```python
from build123d import *

# Parameters (mm, degrees)
EXTRUDE_1_DEPTH     = 3
CUT_EXTRUDE_2_REACH = 76.221
SKETCH_2_R          = 2.1
FILLET_1_R          = 2


with BuildPart() as part:
    # 草图1 → 凸台-拉伸1 (new body)
    with BuildSketch(Plane.XY):
        Polygon((-15, 45.229945154), (15, 45.229945154), (50, -29.684017461), (50, -54.770054846), (-50, -54.770054846), (-50, -29.684017461), align=None)
    extrude(amount=EXTRUDE_1_DEPTH)

    # 草图2 → 切除-拉伸2 (cut, up to next)
    with BuildSketch(Plane.XY.offset(3), mode=Mode.PRIVATE) as cut_extrude_2_sk1:
        with Locations((-9, 35.229945154)):
            Circle(SKETCH_2_R)
    cut_extrude_2_tool1 = extrude(cut_extrude_2_sk1.sketch, amount=-CUT_EXTRUDE_2_REACH, mode=Mode.PRIVATE) & part.part
    # 草图2 → 切除-拉伸2 (cut, up to next)
    with BuildSketch(Plane.XY.offset(3), mode=Mode.PRIVATE) as cut_extrude_2_sk2:
        with Locations((9, 35.229945154)):
            Circle(SKETCH_2_R)
    cut_extrude_2_tool2 = extrude(cut_extrude_2_sk2.sketch, amount=-CUT_EXTRUDE_2_REACH, mode=Mode.PRIVATE) & part.part
    # 草图2 → 切除-拉伸2 (cut, up to next)
    with BuildSketch(Plane.XY.offset(3), mode=Mode.PRIVATE) as cut_extrude_2_sk3:
        with Locations((9, 10.229945154)):
            Circle(SKETCH_2_R)
    cut_extrude_2_tool3 = extrude(cut_extrude_2_sk3.sketch, amount=-CUT_EXTRUDE_2_REACH, mode=Mode.PRIVATE) & part.part
    # 草图2 → 切除-拉伸2 (cut, up to next)
    with BuildSketch(Plane.XY.offset(3), mode=Mode.PRIVATE) as cut_extrude_2_sk4:
        with Locations((-9, 10.229945154)):
            Circle(SKETCH_2_R)
    cut_extrude_2_tool4 = extrude(cut_extrude_2_sk4.sketch, amount=-CUT_EXTRUDE_2_REACH, mode=Mode.PRIVATE) & part.part
    # 草图2 → 切除-拉伸2 (cut, up to next)
    with BuildSketch(Plane.XY.offset(3), mode=Mode.PRIVATE) as cut_extrude_2_sk5:
        with Locations((-20, -36.770054846)):
            Circle(SKETCH_2_R)
    cut_extrude_2_tool5 = extrude(cut_extrude_2_sk5.sketch, amount=-CUT_EXTRUDE_2_REACH, mode=Mode.PRIVATE) & part.part
    # 草图2 → 切除-拉伸2 (cut, up to next)
    with BuildSketch(Plane.XY.offset(3), mode=Mode.PRIVATE) as cut_extrude_2_sk6:
        with Locations((-20, -46.770054846)):
            Circle(SKETCH_2_R)
    cut_extrude_2_tool6 = extrude(cut_extrude_2_sk6.sketch, amount=-CUT_EXTRUDE_2_REACH, mode=Mode.PRIVATE) & part.part
    # 草图2 → 切除-拉伸2 (cut, up to next)
    with BuildSketch(Plane.XY.offset(3), mode=Mode.PRIVATE) as cut_extrude_2_sk7:
        with Locations((20, -46.770054846)):
            Circle(SKETCH_2_R)
    cut_extrude_2_tool7 = extrude(cut_extrude_2_sk7.sketch, amount=-CUT_EXTRUDE_2_REACH, mode=Mode.PRIVATE) & part.part
    # 草图2 → 切除-拉伸2 (cut, up to next)
    with BuildSketch(Plane.XY.offset(3), mode=Mode.PRIVATE) as cut_extrude_2_sk8:
        with Locations((20, -36.770054846)):
            Circle(SKETCH_2_R)
    cut_extrude_2_tool8 = extrude(cut_extrude_2_sk8.sketch, amount=-CUT_EXTRUDE_2_REACH, mode=Mode.PRIVATE) & part.part
    # 草图2 → 切除-拉伸2 (cut, up to next)
    with BuildSketch(Plane.XY.offset(3), mode=Mode.PRIVATE) as cut_extrude_2_sk9:
        with Locations((-9, -14.770054846)):
            Circle(SKETCH_2_R)
    cut_extrude_2_tool9 = extrude(cut_extrude_2_sk9.sketch, amount=-CUT_EXTRUDE_2_REACH, mode=Mode.PRIVATE) & part.part
    # 草图2 → 切除-拉伸2 (cut, up to next)
    with BuildSketch(Plane.XY.offset(3), mode=Mode.PRIVATE) as cut_extrude_2_sk10:
        with Locations((9, -14.770054846)):
            Circle(SKETCH_2_R)
    cut_extrude_2_tool10 = extrude(cut_extrude_2_sk10.sketch, amount=-CUT_EXTRUDE_2_REACH, mode=Mode.PRIVATE) & part.part
    # 草图2 → 切除-拉伸2 (cut, up to next)
    with BuildSketch(Plane.XY.offset(3), mode=Mode.PRIVATE) as cut_extrude_2_sk11:
        with Locations((-35, -36.770054846)):
            Circle(SKETCH_2_R)
    cut_extrude_2_tool11 = extrude(cut_extrude_2_sk11.sketch, amount=-CUT_EXTRUDE_2_REACH, mode=Mode.PRIVATE) & part.part
    # 草图2 → 切除-拉伸2 (cut, up to next)
    with BuildSketch(Plane.XY.offset(3), mode=Mode.PRIVATE) as cut_extrude_2_sk12:
        with Locations((-35, -46.770054846)):
            Circle(SKETCH_2_R)
    cut_extrude_2_tool12 = extrude(cut_extrude_2_sk12.sketch, amount=-CUT_EXTRUDE_2_REACH, mode=Mode.PRIVATE) & part.part
    # 草图2 → 切除-拉伸2 (cut, up to next)
    with BuildSketch(Plane.XY.offset(3), mode=Mode.PRIVATE) as cut_extrude_2_sk13:
        with Locations((35, -36.770054846)):
            Circle(SKETCH_2_R)
    cut_extrude_2_tool13 = extrude(cut_extrude_2_sk13.sketch, amount=-CUT_EXTRUDE_2_REACH, mode=Mode.PRIVATE) & part.part
    # 草图2 → 切除-拉伸2 (cut, up to next)
    with BuildSketch(Plane.XY.offset(3), mode=Mode.PRIVATE) as cut_extrude_2_sk14:
        with Locations((35, -46.770054846)):
            Circle(SKETCH_2_R)
    cut_extrude_2_tool14 = extrude(cut_extrude_2_sk14.sketch, amount=-CUT_EXTRUDE_2_REACH, mode=Mode.PRIVATE) & part.part
    # 草图2 → 切除-拉伸2 (cut, up to next)
    with BuildSketch(Plane.XY.offset(3), mode=Mode.PRIVATE) as cut_extrude_2_sk15:
        with BuildLine():
            Line((-20.314527419, 5.727067103), (-20.314527419, -23.770054846))
            ThreePointArc((-20.314527419, -23.770054846), (-20.607420638, -24.477161627), (-21.314527419, -24.770054846))
            Line((-21.314527419, -24.770054846), (-35.09566023, -24.770054846))
            ThreePointArc((-35.09566023, -24.770054846), (-35.939249041, -24.307044527), (-36.001657204, -23.346770682))
            Line((-36.001657204, -23.346770682), (-22.220524392, 6.150351268))
            ThreePointArc((-22.220524392, 6.150351268), (-21.097729095, 6.703283517), (-20.314527419, 5.727067103))
        make_face()
    cut_extrude_2_tool15 = extrude(cut_extrude_2_sk15.sketch, amount=-CUT_EXTRUDE_2_REACH, mode=Mode.PRIVATE) & part.part
    # 草图2 → 切除-拉伸2 (cut, up to next)
    with BuildSketch(Plane.XY.offset(3), mode=Mode.PRIVATE) as cut_extrude_2_sk16:
        with BuildLine():
            Line((36.001657204, -23.346770682), (22.220524392, 6.150351268))
            ThreePointArc((22.220524392, 6.150351268), (21.097729095, 6.703283517), (20.314527419, 5.727067103))
            Line((20.314527419, 5.727067103), (20.314527419, -23.770054846))
            ThreePointArc((20.314527419, -23.770054846), (20.607420638, -24.477161627), (21.314527419, -24.770054846))
            Line((21.314527419, -24.770054846), (35.09566023, -24.770054846))
            ThreePointArc((35.09566023, -24.770054846), (35.939249041, -24.307044527), (36.001657204, -23.346770682))
        make_face()
    cut_extrude_2_tool16 = extrude(cut_extrude_2_sk16.sketch, amount=-CUT_EXTRUDE_2_REACH, mode=Mode.PRIVATE) & part.part
    add(cut_extrude_2_tool1.solids().sort_by_distance((-9, 35.229945, 3))[0], mode=Mode.SUBTRACT)
    add(cut_extrude_2_tool2.solids().sort_by_distance((9, 35.229945, 3))[0], mode=Mode.SUBTRACT)
    add(cut_extrude_2_tool3.solids().sort_by_distance((9, 10.229945, 3))[0], mode=Mode.SUBTRACT)
    add(cut_extrude_2_tool4.solids().sort_by_distance((-9, 10.229945, 3))[0], mode=Mode.SUBTRACT)
    add(cut_extrude_2_tool5.solids().sort_by_distance((-20, -36.770055, 3))[0], mode=Mode.SUBTRACT)
    add(cut_extrude_2_tool6.solids().sort_by_distance((-20, -46.770055, 3))[0], mode=Mode.SUBTRACT)
    add(cut_extrude_2_tool7.solids().sort_by_distance((20, -46.770055, 3))[0], mode=Mode.SUBTRACT)
    add(cut_extrude_2_tool8.solids().sort_by_distance((20, -36.770055, 3))[0], mode=Mode.SUBTRACT)
    add(cut_extrude_2_tool9.solids().sort_by_distance((-9, -14.770055, 3))[0], mode=Mode.SUBTRACT)
    add(cut_extrude_2_tool10.solids().sort_by_distance((9, -14.770055, 3))[0], mode=Mode.SUBTRACT)
    add(cut_extrude_2_tool11.solids().sort_by_distance((-35, -36.770055, 3))[0], mode=Mode.SUBTRACT)
    add(cut_extrude_2_tool12.solids().sort_by_distance((-35, -46.770055, 3))[0], mode=Mode.SUBTRACT)
    add(cut_extrude_2_tool13.solids().sort_by_distance((35, -36.770055, 3))[0], mode=Mode.SUBTRACT)
    add(cut_extrude_2_tool14.solids().sort_by_distance((35, -46.770055, 3))[0], mode=Mode.SUBTRACT)
    add(cut_extrude_2_tool15.solids().sort_by_distance((-25.803132, -13.304968, 3))[0], mode=Mode.SUBTRACT)
    add(cut_extrude_2_tool16.solids().sort_by_distance((25.803132, -13.304968, 3))[0], mode=Mode.SUBTRACT)

    # 圆角1
    fillet_1_edges = [part.edges().sort_by_distance(p)[0] for p in [
        (-15, 45.229945154, 1.5),
        (-50, -29.684017461, 1.5),
        (-50, -54.770054846, 1.5),
        (50, -54.770054846, 1.5),
        (50, -29.684017461, 1.5),
        (15, 45.229945154, 1.5),
    ]]
    fillet(fillet_1_edges, radius=FILLET_1_R)


solid = part.part
```
Geometry check sheet. Reference: the model listing, model coordinates, mm. A direction names the side the tool comes from. Give positions to 0.01 mm unless a question says otherwise; leave off trailing zeros. Write each loop counter-clockwise with the first axis right and the second up, starting at its lowest first coordinate (ties: lowest second). Pieces come first, ordered by that corner, then holes.
1) Section check B-B, the plane x = -9. Record the boundary of the cut face in (y, z), and give its area (3 significant figures).
2) Access from +Z, -Z, +X, -X, +Y, -Y to the whole of each face (thin tool, end or side, straight path). Record for faces 1 (the flat face through (28, -24.77, 2)), 2 (the flat face through (50, -41, 1)).
3) Section check A-A, the plane y = -3.5. Record the boundary of the cut face in (x, z).
4) Section check C-C, the plane x = -28. Record the boundary of the cut face in (y, z).
5) Gauge pin test, flat ends, axial feed: pin 1 (3.5 mm diameter, centred on x = 20, y = -36.77, fed in from -Z); pin 2 (0.9 mm diameter, centred on y = -12, z = 2, fed in from +X); pin 3 (1.5 mm diameter, centred on x = 27.5, z = 2, fed in from +Y); pin 4 (5.5 mm diameter, centred on x = -9, y = 35.23, fed in from +Z). Record the tip position at first contact, or that the pin passes through.
6) Release check for a two-part mould opening along Y. For faces 3 (the flat face through (1, -15, 3)), 4 (the flat face through (-32.915, 6.884, 1.479)), 5 (the cylindrical face through (6.9, -14.7, 1.5)) record: pulls with the +Y half, pulls with the -Y half, needs draft (parallel to the pull), parting line crosses it, or undercut.
7) Section check D-D, the plane z = 2.4. State how many separate pieces and enclosed holes the cut face has, and give its area (3 significant figures).
8) Material ranges on L1, parallel to Y at x = -9, z = 2.65; L2, parallel to X at y = 9.5, z = 1.2; L3, parallel to Y at x = 34.5, z = 2.4, recorded low to high.
Computed:
1. outline: (-54.77, 0) - (-16.87, 0) - (-16.87, 3) - (-54.77, 3) - close; (-12.67, 0) - (8.13, 0) - (8.13, 3) - (-12.67, 3) - close; (12.33, 0) - (33.13, 0) - (33.13, 3) - (12.33, 3) - close; (37.33, 0) - (45.23, 0) - (45.23, 3) - (37.33, 3) - close
1. area: 262 mm2
2. face 1: +Z, -Z
2. face 2: +Z, -Z, +X, +Y, -Y
3. outline: (-37.77, 0) - (-26.73, 0) - (-26.73, 3) - (-37.77, 3) - close; (-20.31, 0) - (20.31, 0) - (20.31, 3) - (-20.31, 3) - close; (26.73, 0) - (37.77, 0) - (37.77, 3) - (26.73, 3) - close
4. outline: (-54.77, 0) - (-24.77, 0) - (-24.77, 3) - (-54.77, 3) - close; (-6.22, 0) - (17.4, 0) - (17.4, 3) - (-6.22, 3) - close
5. pin 1: passes through
5. pin 2: stops at x = 41.95
5. pin 3: stops at y = 20.08
5. pin 4: stops at z = 3
6. face 3: needs draft
6. face 4: pulls with the +Y half
6. face 5: undercut
7. separate pieces: 1
7. enclosed holes: 16
7. area: 6,620 mm2
8. L1: y = -54.77 to -16.87, -12.67 to 8.13, 12.33 to 33.13, 37.33 to 45.23
8. L2: x = -31.69 to -10.97, -7.03 to 7.03, 10.97 to 31.69
8. L3: y = -54.77 to -48.81, -44.73 to -38.81, -34.73 to -24.77, -20.13 to 3.49
